For this review, take the finished solid that the model builds, in its own axes (mm). Round coordinates to 2 decimals unless told otherwise and drop trailing zeros. Loops run counter-clockwise (first coordinate to the right, second up) from the corner with the lowest first, then second, coordinate; pieces in that order, holes last.
1. Clearance check with flat-ended pins moving along their axes: pin 1 Ø5 at (x, z) = (387, -1.5) entering from -Y; pin 2 Ø5 at (x, y) = (111.5, -0.5) entering from +Z; pin 3 Ø2 at (x, y) = (230.5, 3.5) entering from +Z. State where each tip first meets the part, or that it passes through.
2. To check wall thickness, follow line 1 along X through (y, z) = (5, 0.5); line 2 along Z through (x, y) = (157, -2.25); line 3 along Z through (x, y) = (410.5, -0.5). State the ranges of each line that lie inside material, in increasing order.
3. Consider section B-B on x = 222. State the section outline as (y, z) points.
4. Consider section A-A on z = 0. State the section outline as (x, y) points.
from build123d import *

# Parameters (mm, degrees)
CUT_EXTRUDE_1_DEPTH      = 3
CUT_EXTRUDE_1_DEPTH_BACK = 3


with BuildPart() as part:
    # Sketch 1 → Revolve 1 (revolve)
    with BuildSketch(Plane.XY, mode=Mode.PRIVATE) as revolve_1_sk:
        Polygon((0, 0), (0, 3.233), (0.767, 4), (467, 4), (467, 9.75), (489, 9.75), (489, 0), align=None)
    revolve(revolve_1_sk.sketch.rotate(Axis((489, 0, 0), (-1, 0, 0)), 270), axis=Axis((489, 0, 0), (-1, 0, 0)))

    # Sketch 2 → Cut-Extrude 1 (cut, two sides: drawn at the far end of the back side and taken through both)
    with BuildSketch(Plane(origin=(0, 0, 0), x_dir=(1, 0, 0), z_dir=(0, 1, 0)).offset(-CUT_EXTRUDE_1_DEPTH_BACK)):
        Polygon((-5, -12), (35.4, -12), (26.4, -3), (20, -3), (18, -5), (18, -10), (-3, -10), (-3, 10), (18, 10), (18, 5), (20, 3), (26.4, 3), (35.4, 12), (-5, 12), align=None)
    extrude(amount=CUT_EXTRUDE_1_DEPTH + CUT_EXTRUDE_1_DEPTH_BACK, mode=Mode.SUBTRACT)


solid = part.part
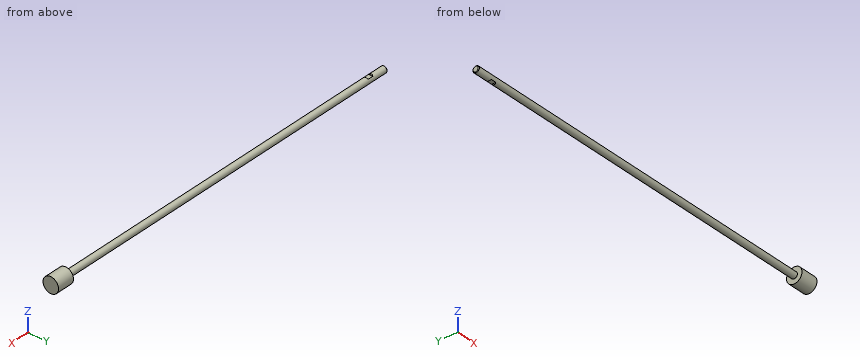
Resolved:
1. pin 1: stops at y = -4
1. pin 2: stops at z = 4
1. pin 3: stops at z = 3.12
2. line 1: x = 467 to 489
2. line 2: z = -3.31 to 3.31
2. line 3: z = -3.97 to 3.97
3. outline: circle Ø8 at (0, 0)
4. outline: (0, -3.23) - (0.77, -4) - (467, -4) - (467, -9.75) - (489, -9.75) - (489, 9.75) - (467, 9.75) - (467, 4) - (0.77, 4) - (0, 3.23) - close
